Verification items for the finished model (mm, model axes). A direction names the side the tool comes from. Give positions to 0.01 mm unless a question says otherwise; leave off trailing zeros. Write each loop counter-clockwise with the first axis right and the second up, starting at its lowest first coordinate (ties: lowest second). Pieces come first, ordered by that corner, then holes. Notation, with made-up numbers: (-12.5, 21) - (-4.5, 21) arc R28 cw to (-4.5, 49) - close; hole circle Ø3 at (85.25, 16.5). An arc over 180 degrees is marked (long way). Put each result on its own line as item: value.
from build123d import *

# Parameters (mm, degrees)
SKETCH_1_W                    = 20
SKETCH_1_H                    = 16
EXTRUDE_1_DEPTH               = 11.5
CUT_EXTRUDE_1_DEPTH           = 25.916109247
SKETCH_3_W                    = 3.3
SKETCH_3_H                    = 16
HOLE_WIZARD_5_0_5_1_D         = 5
SKETCH_6_W                    = 0.8
SKETCH_6_H                    = 3
HOLE_WIZARD_2_4_2_4_1_D       = 2.4
HOLE_WIZARD_2_4_2_4_1_DEPTH   = 11.5
HOLE_WIZARD_2_05_2_05_1_D     = 2.05
HOLE_WIZARD_2_05_2_05_1_DEPTH = 4.5
HOLE_WIZARD_2_05_2_05_1_TIP   = 0.615882135
M2X0_41_D                     = 1
M2X0_41_DEPTH                 = 4.5
M2X0_41_CBORE_D               = 2
M2X0_41_CBORE_DEPTH           = 2
CHAMFER_1_SIZE                = 0.2


with BuildPart() as part:
    # Эскиз1 → Бобышка-Вытянуть1 (new body)
    with BuildSketch(Plane(origin=(0, 0, 0), x_dir=(-1, 0, 0), z_dir=(0, 0, -1))):
        with Locations((-5.25, 0)):
            Rectangle(SKETCH_1_W, SKETCH_1_H)
    extrude(amount=-EXTRUDE_1_DEPTH)

    # Эскиз2 → Вырез-Вытянуть1 (cut, through all)
    with BuildSketch(Plane(origin=(0, 8, 0), x_dir=(-1, 0, 0), z_dir=(0, 1, 0))):
        with BuildLine():
            Line((-15.25, 8.5), (-15.25, 6.5))
            Line((-15.25, 6.5), (-9.894837039, 6.5))
            ThreePointArc((-9.894837039, 6.5), (-10.05, 7.5), (-9.894837039, 8.5))
            Line((-9.894837039, 8.5), (-15.25, 8.5))
        make_face()
    extrude(amount=-CUT_EXTRUDE_1_DEPTH, mode=Mode.SUBTRACT)

    # Эскиз3 → Вырез-Повернуть1 (revolve, cut)
    with BuildSketch(Plane.XY.offset(7.5)):
        with Locations((8.4, 0)):
            Rectangle(SKETCH_3_W, SKETCH_3_H)
    revolve(axis=Axis((6.75, 8, 7.5), (0, -1, 0)), mode=Mode.SUBTRACT)

    # Диаметр отверстия Ø5.0 (5)1 (through all)
    with Locations(Plane(origin=(0, 0, 0), x_dir=(-1, 0, 0), z_dir=(0, 0, -1))):
        with Locations((0, 0)):
            Hole(HOLE_WIZARD_5_0_5_1_D / 2)

    # Эскиз6 → Диаметр отверстия Ø1.6 (1.6)1 (revolve, cut)
    with BuildSketch(Plane(origin=(13.25, 0, 8.5), x_dir=(0, 1, 0), z_dir=(1, 0, 0))):
        with Locations((0.4, 1.5)):
            Rectangle(SKETCH_6_W, SKETCH_6_H)
    revolve(axis=Axis((13.25, 0, 2.15), (0, 0, 1)), mode=Mode.SUBTRACT)

    # Диаметр отверстия Ø2.4 (2.4)1
    with Locations(Plane(origin=(0, 0, 0), x_dir=(-1, 0, 0), z_dir=(0, 0, -1))):
        with Locations((-13.25, 0)):
            Hole(HOLE_WIZARD_2_4_2_4_1_D / 2, depth=HOLE_WIZARD_2_4_2_4_1_DEPTH)

    # Диаметр отверстия Ø2.05 (2.05)1
    with Locations(Plane(origin=(0, -8, 0), x_dir=(-1, 0, 0), z_dir=(0, -1, 0))):
        with Locations((1.25, -6.5)):
            Hole(HOLE_WIZARD_2_05_2_05_1_D / 2, depth=HOLE_WIZARD_2_05_2_05_1_DEPTH)
            with Locations((0, 0, -(HOLE_WIZARD_2_05_2_05_1_DEPTH + HOLE_WIZARD_2_05_2_05_1_TIP / 2))):  # 118° drill point
                Cone(0, HOLE_WIZARD_2_05_2_05_1_D / 2, HOLE_WIZARD_2_05_2_05_1_TIP, mode=Mode.SUBTRACT)

    # Отверстие обработанное метчиком M2x0.41
    with Locations(Plane(origin=(0, -8, 0), x_dir=(-1, 0, 0), z_dir=(0, -1, 0))):
        with Locations((2.25, -9)):
            CounterBoreHole(M2X0_41_D / 2, M2X0_41_CBORE_D / 2, M2X0_41_CBORE_DEPTH, depth=M2X0_41_DEPTH)

    # Фаска1
    chamfer_1_edges = [part.edges().sort_by_distance(p)[0] for p in [
        (-4.75, 0, 11.5),
        (5.25, 8, 11.5),
        (15.25, -8, 3.25),
        (15.25, 8, 3.25),
        (15.25, 0, 11.5),
        (5.25, 8, 0),
        (-4.75, 0, 0),
        (5.25, -8, 0),
        (15.25, 0, 0),
        (5.25, -8, 11.5),
        (15.25, 8, 10),
        (-4.75, 8, 5.75),
        (-4.75, -8, 5.75),
        (15.25, -8, 10),
    ]]
    chamfer(chamfer_1_edges, length=CHAMFER_1_SIZE)


solid = part.part
Q1. Section check D-D, the plane z = 4.75. Record the cut outline in (x, y).
Answers follow:
outline: (-4.75, -7.8) - (-4.55, -8) - (4.93, -8) - (4.93, 8) - (-4.55, 8) - (-4.75, 7.8) - close; (8.57, -8) - (15.05, -8) - (15.25, -7.8) - (15.25, 7.8) - (15.05, 8) - (8.57, 8) - close; hole circle Ø5 at (0, 0); hole circle Ø2.4 at (13.25, 0)
Q2. Release check for a two-part mould opening along Z. For faces 4 (the face through (15.25, 0, 3)), 5 (the face through (11, 0, 6.5)), 6 (the face through (5, 0, 11.5)) record: released by +Z, released by -Z, zero draft, split by the parting line, or undercut.
Answers follow:
face 4: zero draft
face 5: undercut
face 6: released by +Z
Q3. Section check C-C, the plane y = 3. Record the cut outline in (x, z).
Answers follow:
outline: (-4.75, 0.2) - (-4.55, 0) - (15.05, 0) - (15.25, 0.2) - (15.25, 6.5) - (9.89, 6.5) arc R3.3 cw (long way) to (9.89, 8.5) - (15.25, 8.5) - (15.25, 11.3) - (15.05, 11.5) - (-4.55, 11.5) - (-4.75, 11.3) - close
Q4. Scan lines: line 1 along Z through (x, y) = (14.75, 2); line 2 along Y through (x, z) = (0, 7); line 3 along Z through (x, y) = (-1.25, -4.75) (3 decimals). Record each from-to range of solid material in increasing order.
Answers follow:
line 1: z = 0 to 6.5, 8.5 to 11.5
line 2: y = -8 to -2.5, 2.5 to 8
line 3: z = 0 to 5.475, 7.525 to 11.5
Q5. Go/stop test with flat-tipped pins: pin 1 Ø8 at (x, y) = (0, 0) entering from +Z; pin 2 Ø1.4 at (x, y) = (13.25, 0) entering from +Z. Record where each tip stops, or that it passes through.
Answers follow:
pin 1: stops at z = 11.5
pin 2: passes through
Q6. Section check B-B, the plane z = 2. Record the cut outline in (x, y), plus the area to 3 significant figures.
Answers follow:
outline: (-4.75, -7.8) - (-4.55, -8) - (15.05, -8) - (15.25, -7.8) - (15.25, 7.8) - (15.05, 8) - (-4.55, 8) - (-4.75, 7.8) - close; hole circle Ø5 at (0, 0); hole circle Ø2.4 at (13.25, 0)
area: 296 mm2
Q7. Set-up check for faces 1 (the face through (-2, -3.5, 9)), 2 (the face through (14.395, 0.36, 3.296)), 3 (the face through (11.9, 0.1, 8.5)): record each of +Z, -Z, +X, -X, +Y, -Y from which the full face is reachable in a straight line by a thin tool's end or side.
Answers follow:
face 1: -Y
face 2: +Z, -Z
face 3: +X, +Y, -Y
Q8. Section check A-A, the plane x = 0. Record the cut outline in (y, z), plus the area to 3 significant figures.
Answers follow:
outline: (-8, 0.2) - (-7.8, 0) - (-2.5, 0) - (-2.5, 11.5) - (-7.8, 11.5) - (-8, 11.3) - close; (2.5, 0) - (7.8, 0) - (8, 0.2) - (8, 11.3) - (7.8, 11.5) - (2.5, 11.5) - close
area: 126 mm2
